Could you check a few things on this model? Use its own coordinates, in mm. A direction names the side the tool comes from. Give positions to 0.01 mm unless a question says otherwise; leave off trailing zeros. Loops run counter-clockwise (first coordinate to the right, second up) from the corner with the lowest first, then second, coordinate; pieces in that order, holes last. Notation, with made-up numbers: (81, -10) - (118, -10) arc R11 ccw to (118, 2) - close; hole circle Ø4 at (-35, 61.5). An arc over 180 degrees is marked (long way). Use CSV: the item, a comma, the result in double quotes.
from build123d import *

# Parameters (mm, degrees)
F0_W     = 34
F0_H     = 40
F0_R     = 0.5
F0_W_2   = 3
F1_DEPTH = 3
F2_R     = 1
F3_DEPTH = 3


with BuildPart() as f1:
    # F0 (on Top) → F1 (new body)
    with BuildSketch(Plane.XY):
        with Locations((20, 20)):
            Rectangle(F0_W, F0_H)
        with BuildLine():
            ThreePointArc((27.25, 10), (24.68934, 8.93934), (25.75, 11.5))
            ThreePointArc((25.75, 11.5), (26.81066, 11.06066), (27.25, 10))
        make_face(mode=Mode.SUBTRACT)
        with Locations((6.5, 30)):
            Circle(F0_R, mode=Mode.SUBTRACT)
        Polygon((8.75, 23.75), (8.75, 36.25), (31.75, 36.25), (31.75, 23.75), (25.75, 23.75), (14.75, 23.75), align=None, mode=Mode.SUBTRACT)
        with Locations((34, 30)):
            Circle(F0_R, mode=Mode.SUBTRACT)
        with Locations((1.5, 20)):
            Rectangle(F0_W_2, F0_H)
    extrude(amount=F1_DEPTH)

    # F2 (on Right) → F3 (join)
    with BuildSketch(Plane.YZ):
        Polygon((0, 3), (0, 0), (20, 0), (40, 0), (40, 30), (40, 33), (34, 33), (0, 33), align=None)
        with BuildLine():
            ThreePointArc((21, 8.875), (20.707107, 8.167893), (20, 7.875))
            ThreePointArc((20, 7.875), (19, 8.875), (20, 9.875))
            ThreePointArc((20, 9.875), (20.707107, 9.582107), (21, 8.875))
        make_face(mode=Mode.SUBTRACT)
        with Locations((9.875, 18)):
            Circle(F2_R, mode=Mode.SUBTRACT)
        with BuildLine():
            ThreePointArc((23.5, 18), (22.474874, 15.525126), (20, 14.5))
            ThreePointArc((20, 14.5), (17.525126, 15.525126), (16.5, 18))
            ThreePointArc((16.5, 18), (17.525126, 20.474874), (20, 21.5))
            ThreePointArc((20, 21.5), (22.474874, 20.474874), (23.5, 18))
        make_face(mode=Mode.SUBTRACT)
        with BuildLine():
            ThreePointArc((31.125, 18), (30.125, 17), (29.125, 18))
            ThreePointArc((29.125, 18), (30.125, 19), (31.125, 18))
        make_face(mode=Mode.SUBTRACT)
        with BuildLine():
            ThreePointArc((21, 27.125), (20.707107, 26.417893), (20, 26.125))
            ThreePointArc((20, 26.125), (19.292893, 27.832107), (21, 27.125))
        make_face(mode=Mode.SUBTRACT)
    extrude(amount=F3_DEPTH)


solid = f1.part
1) Suppose I cut it at B-B (y = 34). Please give me the cut outline in (x, z).
Answer below:
outline,"(0, 0) - (8.75, 0) - (8.75, 3) - (3, 3) - (3, 33) - (0, 33) - close; (31.75, 0) - (37, 0) - (37, 3) - (31.75, 3) - close"
2) Suppose I cut it at A-A (x = 22.5). Please give me the cut outline in (y, z).
Answer below:
outline,"(0, 0) - (23.75, 0) - (23.75, 3) - (0, 3) - close; (36.25, 0) - (40, 0) - (40, 3) - (36.25, 3) - close"
3) We'd pull the mould along X, two halves only. Please class faces 4 (the flat face through (12, 0, 2)), 5 (the flat face through (3, 20, 22)), 6 (the flat face through (20, 36.25, 1)): +X half, -X half, draft (parallel to the pull), parting line (faces both ways), or undercut.
Answer below:
face 4,"draft"
face 5,"+X half"
face 6,"undercut"
4) Suppose I cut it at C-C (y = 13). Please give me the cut outline in (x, z).
Answer below:
outline,"(0, 0) - (37, 0) - (37, 3) - (3, 3) - (3, 33) - (0, 33) - close"
5) I'm going to push flat-ended pins straight in: P1, Ø1.8, axis at y = 9.875, z = 18, coming from the -X side; P2, Ø2, axis at y = 9.5, z = 6, coming from the -X side; P3, Ø2, axis at y = 6.5, z = 9.5, coming from the +X side. Where does each tip first touch, or does it pass through?
Answer below:
P1,"passes through"
P2,"stops at x = 0"
P3,"stops at x = 3"
6) I need wall thicknesses on line 1 along Z through (x, y) = (1.65, 20) (3 decimals); line 2 along X through (y, z) = (10, 1.7); line 3 along X through (y, z) = (34, 28). Which ranges of each line are inside material? Lowest first, please.
Answer below:
line 1,"z = 0 to 7.875, 9.875 to 14.5, 21.5 to 26.125, 28.125 to 33"
line 2,"x = 0 to 24.25, 27.25 to 37"
line 3,"x = 0 to 3"
7) Which directions (+Z, -Z, +X, -X, +Y, -Y) give clear straight access to the entire face, cutting with the end or side of a thin tool? Please do faces 1 (the flat face through (20, 16, 3)), 2 (the flat face through (37, 20, 1)), 3 (the flat face through (20, 23.75, 1)).
Answer below:
face 1,"+Z, +X, +Y, -Y"
face 2,"+Z, -Z, +X, +Y, -Y"
face 3,"+Z, -Z"
8) Suppose I cut it at D-D (z = 23). Please give me the cut outline in (x, y), plus the area to 3 significant figures.
Answer below:
outline,"(0, 0) - (3, 0) - (3, 40) - (0, 40) - close"
area,"120 mm2"
